from build123d import *

# Parameters (mm, degrees)
BOSS_EXTRUDE1_DEPTH = 7.9375
SKETCH3_R           = 6.429375
CUT_EXTRUDE1_DEPTH  = 0.49609375
CUT_EXTRUDE1_DRAFT  = -45
CHAMFER1_SIZE       = 1.190625


# Read off the part's stored shape, not the designer's step: Cut-Extrude2
with BuildPart() as part:
    # Sketch1 → Revolve1 (revolve)
    with BuildSketch(Plane(origin=(0, 0, 0), x_dir=(0, 0, -1), z_dir=(1, 0, 0))):
        Polygon((9.921875, 4.7625), (41.671875, 4.7625), (41.671875, 0), (0, 0), (0, 7.14375), (7.9375, 7.14375), (7.9375, 10.31875), (9.921875, 10.31875), align=None)
    revolve(axis=Axis((0, 0, -41.671875), (0, 0, 1)))

    # Sketch2 → Boss-Extrude1 (add)
    with BuildSketch(Plane.XY):
        Polygon((7.14375, 4.124445986), (0, 8.248891971), (-7.14375, 4.124445986), (-7.14375, -4.124445986), (0, -8.248891971), (7.14375, -4.124445986), align=None)
    extrude(amount=-BOSS_EXTRUDE1_DEPTH)

    # Cut-Extrude2 outline → Cut-Extrude2 (revolve, cut)
    with BuildSketch(Plane.XZ):
        Polygon((8.248891975, 1.48e-06), (7.143748081, 1.48e-06), (8.248891975, -0.638054017), align=None)
    revolve(axis=Axis((0, 0, 0), (0, 0, 1)), mode=Mode.SUBTRACT)


with BuildPart() as cut_extrude1_tool:
    # Sketch3 → Cut-Extrude1 (with draft: the straight prism first)
    with BuildSketch(Plane.XY):
        Circle(SKETCH3_R)
    extrude(amount=-CUT_EXTRUDE1_DEPTH)
    # Cut-Extrude1: the draft: its side faces are tilted about the plane it starts from
    cut_extrude1_sides = [cut_extrude1_tool.faces().sort_by_distance(p)[0] for p in [
        (-6.429375, 0, -0.248046875),
    ]]
    draft(cut_extrude1_sides, Plane.XY, CUT_EXTRUDE1_DRAFT)


with BuildPart() as part_1:
    add(part.part)

    # Cut-Extrude1: cut by cut_extrude1_tool
    add(cut_extrude1_tool.part, mode=Mode.SUBTRACT)

    # Chamfer1
    chamfer1_edges = [part_1.edges().sort_by_distance(p)[0] for p in [
        (0, -4.7625, -41.671875),
    ]]
    chamfer(chamfer1_edges, length=CHAMFER1_SIZE)


solid = part_1.part
CAD build for the part. Positions are in the model's coordinates, mm. A direction names the side the tool comes from. Coordinates: 2 decimals unless noted, no trailing zeros. Write each loop counter-clockwise with the first axis right and the second up, starting at its lowest first coordinate (ties: lowest second). Pieces come first, ordered by that corner, then holes. Notation, with made-up numbers: M -23.75,20 L -5.75,20 A21 ccw -5.75,59 Z; hole C 21,32.5 d10. An arc over 180 degrees is marked long. Answer as a JSON object with one key per item and string values. Group by question number.
1) Pin check, flat tips, straight feed: pin 1 Ø3 at (x, z) = (-1.5, -21.5) entering from +Y; pin 2 Ø6.5 at (y, z) = (-0.5, -4) entering from -X; pin 3 Ø4 at (x, z) = (-0.5, -5.5) entering from -Y. Stop position of each tip, or through.
2) Saw through at A-A (z = -7.5). Write the cut outline in (x, y), plus the area to 3 significant figures.
3) Saw through at B-B (z = -33). Write the cut outline in (x, y) (1 decimal), plus the area to 3 significant figures.
4) Wall check: line 1 (X direction, y = -0.25, z = -5); line 2 (Z direction, x = -7.5, y = 0.5); line 3 (Z direction, x = 5.75, y = 3.25). Give the ranges that are in metal, low to high. Write a range as from..to.
5) Tool access for faces 5 (the face through (-7.144, 0, -4)), 6 (the face through (-2.44, 7.02, -7.938)), 7 (the face through (-3.62, -6.16, -3.91)): list every direction of +Z, -Z, +X, -X, +Y, -Y with a clear straight run to the whole face (end or side of a thin tool).
6) Mould opens along X. For faces 1 (the face through (0, 0, -0.496)), 2 (the face through (4.44, 2.15, -9.922)), 3 (the face through (-6.37, 3.7, -0.13)), 4 (the face through (3.522, -6.216, -3.913)) say: +X half, -X half, draft (parallel to the pull), parting line (faces both ways), or undercut.
Values follow:
{
 "1": {"pin 1": "stops at y = 4.76", "pin 2": "stops at x = -7.14", "pin 3": "stops at y = -8.25"},
 "2": {"outline": "M -7.14,-4.12 L 0,-8.25 L 7.14,-4.12 L 7.14,4.12 L 0,8.25 L -7.14,4.12 Z", "area": "177 mm2"},
 "3": {"outline": "C 0,0 d9.5", "area": "71.3 mm2"},
 "4": {"line 1": "x = -7.14..7.14", "line 2": "z = -9.92..-7.94", "line 3": "z = -9.92..0"},
 "5": {"face 5": "+Z, -X, +Y, -Y", "face 6": "+Z", "face 7": "+Z, -X, -Y"},
 "6": {"face 1": "undercut", "face 2": "draft", "face 3": "-X half", "face 4": "+X half"}
}
